Model file for the job. Use its own axes, mm. A direction names the side the tool comes from. Coordinates: 2 decimals unless noted, no trailing zeros. Write each loop counter-clockwise with the first axis right and the second up, starting at its lowest first coordinate (ties: lowest second). Pieces come first, ordered by that corner, then holes. Notation, with made-up numbers: M 50.25,53 L 80.25,53 A22 ccw 80.25,65 Z; hole C 54.5,74 d11. An arc over 180 degrees is marked long. Use CSV: the item, a comma, the result in double quotes. Start each with the question number.
from build123d import *

# Parameters (mm, degrees)
EXTRUDE_1_DEPTH      = 36
EXTRUDE_START        = -2
EXTRUDE_2_DEPTH      = 2
SKETCH_3_R           = 2.5
SKETCH_3_R_2         = 1.5
CUT_EXTRUDE_1_DEPTH  = 126.677663072
EXTRUDE_3_DEPTH      = 2
EXTRUDE_3_DEPTH_BACK = 2
SKETCH_4_R           = 1.5
SKETCH_5_W           = 98.68516208
SKETCH_5_H           = 47.907231557
CUT_EXTRUDE_2_DEPTH  = 133.268193437
SKETCH_6_R           = 1.5
EXTRUDE_4_DEPTH      = 3


with BuildPart() as part:
    # Sketch 1 → Extrude 1 (new body)
    with BuildSketch(Plane(origin=(0, 0, 0), x_dir=(1, 0, 0), z_dir=(0, 1, 0))):
        with BuildLine():
            Line((3, -79.943730211), (3, -89.993749756))
            Line((3, -89.993749756), (1, -89.993749756))
            Line((1, -89.993749756), (1, -54.990908339))
            ThreePointArc((1, -54.990908339), (55, 0), (1, 54.990908339))
            Line((1, 54.990908339), (1, 79.993749756))
            Line((1, 79.993749756), (1, 89.993749756))
            Line((1, 89.993749756), (3, 89.993749756))
            Line((3, 89.993749756), (3, 79.943730211))
            ThreePointArc((3, 79.943730211), (80, 0), (3, -79.943730211))
        make_face()
        with BuildLine():
            Line((3, 77.441913716), (3, 57.421685799))
            ThreePointArc((3, 57.421685799), (57.5, 0), (3, -57.421685799))
            Line((3, -57.421685799), (3, -77.441913716))
            ThreePointArc((3, -77.441913716), (77.5, 0), (3, 77.441913716))
        make_face(mode=Mode.SUBTRACT)
    extrude(amount=EXTRUDE_1_DEPTH)

    # Sketch 2 → Extrude 2 (add)
    with BuildSketch(Plane(origin=(0, 0, 0), x_dir=(1, 0, 0), z_dir=(0, 1, 0)).offset(EXTRUDE_START)):
        with BuildLine():
            Line((1, 89.993749756), (1, 54.990908339))
            ThreePointArc((1, 54.990908339), (55, 0), (1, -54.990908339))
            Line((1, -54.990908339), (1, -89.993749756))
            Line((1, -89.993749756), (3, -89.993749756))
            Line((3, -89.993749756), (3, -79.943730211))
            ThreePointArc((3, -79.943730211), (80, 0), (3, 79.943730211))
            Line((3, 79.943730211), (3, 89.993749756))
            Line((3, 89.993749756), (1, 89.993749756))
        make_face()
    extrude(amount=EXTRUDE_2_DEPTH)

    # Sketch 3 → Cut-Extrude 1 (cut, through all)
    with BuildSketch(Plane(origin=(0, 0, 0), x_dir=(0, 0, -1), z_dir=(1, 0, 0))):
        with Locations(Location((-84.968739983, 30, 0), (0, 0, 180))):
            Circle(SKETCH_3_R)
        with Locations(Location((-84.968739983, 17, 0), (0, 0, 180))):
            Circle(SKETCH_3_R_2)
        with Locations(Location((84.968739983, 17, 0), (0, 0, 180))):
            Circle(SKETCH_3_R_2)
        with Locations(Location((84.968739983, 30, 0), (0, 0, 180))):
            Circle(SKETCH_3_R)
        with Locations(Location((-84.968739983, 4, 0), (0, 0, 180))):
            Circle(SKETCH_3_R)
    extrude(amount=CUT_EXTRUDE_1_DEPTH, mode=Mode.SUBTRACT)

    # Sketch 4 → Extrude 3 (add, two sides: drawn at the far end of the back side and taken through both)
    with BuildSketch(Plane.XY.offset(-EXTRUDE_3_DEPTH_BACK)):
        Polygon((80, 36), (55, 36), (55, -2), (80, -2), (90, -2), (90, 36), align=None)
        with Locations((85, 17)):
            Circle(SKETCH_4_R, mode=Mode.SUBTRACT)
    extrude(amount=EXTRUDE_3_DEPTH + EXTRUDE_3_DEPTH_BACK)

    # Sketch 5 → Cut-Extrude 2 (cut, through all)
    with BuildSketch(Plane.XY):
        with Locations((47.157910723, 20.571893337)):
            Rectangle(SKETCH_5_W, SKETCH_5_H)
    extrude(amount=-CUT_EXTRUDE_2_DEPTH, mode=Mode.SUBTRACT)

    # Sketch 6 → Extrude 4 (add)
    with BuildSketch(Plane(origin=(0, 36, 0), x_dir=(1, 0, 0), z_dir=(0, 1, 0))):
        with BuildLine():
            Line((58.650074089, -54.407433402), (54.407433402, -58.650074089))
            Line((54.407433402, -58.650074089), (56.882307136, -61.124947823))
            ThreePointArc((56.882307136, -61.124947823), (61.124947823, -61.124947823), (61.124947823, -56.882307136))
            Line((61.124947823, -56.882307136), (58.650074089, -54.407433402))
        make_face()
        with Locations(Location((59.003627479, -59.003627479, 0), (0, 0, 270))):
            Circle(SKETCH_6_R, mode=Mode.SUBTRACT)
    extrude(amount=-EXTRUDE_4_DEPTH)


solid = part.part
1) Drop flat-ended pins along their axis: P1, Ø4, axis at x = 59, z = 59, coming from the -Y side; P2, Ø11, axis at x = 86.5, y = 24, coming from the +Z side; P3, Ø8.5, axis at x = 57.5, z = 59.5, coming from the -Y side; P4, Ø5, axis at y = 17, z = 84.97, coming from the +X side. Give the stop position or say it passes through.
2) Band-saw the part on D-D on x = 13.5. List the corners of the cut face in (y, z), then the cut area to 3 significant figures.
3) Band-saw the part on B-B on x = 85. List the corners of the cut face in (y, z), then the cut area to 3 significant figures.
4) Band-saw the part on A-A on y = 30. List the corners of the cut face in (x, z) (3 decimals).
5) Band-saw the part on C-C on y = 17. List the corners of the cut face in (x, z) (3 decimals), then the cut area to 3 significant figures.
6) Tool access for faces 5 (the face through (55.63, 34.52, 59.87)), 6 (the face through (59.9, 34.52, 55.66)), 7 (the face through (3, 17, 87)): list every direction of +Z, -Z, +X, -X, +Y, -Y with a clear straight run to the whole face (end or side of a thin tool).
7) Wall check: L1, parallel to Y at x = 85, z = 0.7; L2, parallel to X at y = 16.5, z = 50.5; L3, parallel to X at y = 11, z = 43. Give the ranges that are in metal, low to high. Write a range as [from, to].
8) Two-plate mould, pull along X, no slides. Class faces 1 (the face through (60.27, 34.52, 59.81)), 2 (the face through (61.08, 34.52, 61.17)), 3 (the face through (90, 17, 1)), 4 (the face through (87, 17, 2)): pulls with the +X half, pulls with the -X half, needs draft (parallel to the pull), parting line crosses it, or undercut.
Findings below:
1,P1,"stops at y = 33"
1,P2,"stops at z = 2"
1,P3,"stops at y = -2"
1,P4,"stops at x = 3"
2,outline,"M -2,53.32 L 36,53.32 L 36,55.89 L 0,55.89 L 0,76.32 L 36,76.32 L 36,78.85 L -2,78.85 Z"
2,area,"235 mm2"
3,outline,"M -2,0 L 15.5,0 L 15.5,2 L -2,2 Z; M 18.5,0 L 36,0 L 36,2 L 18.5,2 Z"
3,area,"70.0 mm2"
4,outline,"M 1,54.991 A55 cw 55,0 L 90,0 L 90,2 L 79.975,2 A80 ccw 3,79.944 L 3,82.469 L 1,82.469 Z; M 1,87.469 L 3,87.469 L 3,89.994 L 1,89.994 Z; hole M 3,57.422 A57.5 cw 57.465,2 L 77.474,2 A77.5 ccw 3,77.442 Z"
5,outline,"M 1,54.991 A55 cw 55,0 L 83.5,0 L 83.5,2 L 79.975,2 A80 ccw 3,79.944 L 3,83.469 L 1,83.469 Z; M 1,86.469 L 3,86.469 L 3,89.994 L 1,89.994 Z; M 86.5,0 L 90,0 L 90,2 L 86.5,2 Z; hole M 3,57.422 A57.5 cw 57.465,2 L 77.474,2 A77.5 ccw 3,77.442 Z"
5,area,"633 mm2"
6,face 5,"+Z, +Y, -Y"
6,face 6,"+X, +Y, -Y"
6,face 7,"+Z, +X, +Y, -Y"
7,L1,"y = [-2, 15.5], [18.5, 36]"
7,L2,"x = [21.79, 27.5], [58.79, 62.05]"
7,L3,"x = [34.29, 38.17], [64.48, 67.46]"
8,face 1,"undercut"
8,face 2,"undercut"
8,face 3,"pulls with the +X half"
8,face 4,"needs draft"
